from build123d import *

# Parameters (mm, degrees)
SKETCH1_W              = 25
SKETCH1_H              = 35
SKETCH1_R              = 3.45
SKETCH1_R_2            = 1.5
BOSS_EXTRUDE1_DEPTH    = 13
SKETCH5_W              = 21
SKETCH5_H              = 31
CUT_EXTRUDE1_DEPTH     = 11
CUT_EXTRUDE2_REACH     = 41.373
SKETCH7_R              = 2.5
BOSS_EXTRUDE3_DEPTH    = 13
SKETCH11_R             = 3.25
CUT_EXTRUDE4_DEPTH     = 12
CUT_EXTRUDE5_START     = 12
CUT_EXTRUDE5_OUTLINE_R = 1.75
CUT_EXTRUDE5_DEPTH     = 1


# Read off the part's stored shape, not the designer's step: Cut-Extrude5
with BuildPart() as part:
    # Sketch1 → Boss-Extrude1 (new body)
    with BuildSketch(Plane(origin=(0, 0, 0), x_dir=(1, 0, 0), z_dir=(0, 1, 0))):
        with Locations((0, -7.840328725)):
            Rectangle(SKETCH1_W, SKETCH1_H)
        with Locations(Location((0, 0, 0), (0, 0, 90))):
            Circle(SKETCH1_R, mode=Mode.SUBTRACT)
        with Locations(Location((8.5, 0, 0), (0, 0, 90))):
            Circle(SKETCH1_R_2, mode=Mode.SUBTRACT)
    extrude(amount=BOSS_EXTRUDE1_DEPTH)

    # Sketch5 → Cut-Extrude1 (cut)
    with BuildSketch(Plane(origin=(0, 13, 0), x_dir=(1, 0, 0), z_dir=(0, 1, 0))):
        with Locations((0, -7.840328725)):
            Rectangle(SKETCH5_W, SKETCH5_H)
    extrude(amount=-CUT_EXTRUDE1_DEPTH, mode=Mode.SUBTRACT)

    # Sketch7 → Cut-Extrude2 (cut, up to next)
    with BuildSketch(Plane.XY.offset(25.340328725), mode=Mode.PRIVATE) as cut_extrude2_sk1:
        with Locations((0, 7)):
            Circle(SKETCH7_R)
    cut_extrude2_tool1 = extrude(cut_extrude2_sk1.sketch, amount=-CUT_EXTRUDE2_REACH, mode=Mode.PRIVATE) & part.part
    add(cut_extrude2_tool1.solids().sort_by_distance((0, 7, 25.340329))[0], mode=Mode.SUBTRACT)

    # Sketch9 → Boss-Extrude3 (add, through all)
    with BuildSketch(Plane(origin=(0, 13, 0), x_dir=(1, 0, 0), z_dir=(0, 1, 0))):
        with BuildLine():
            Line((-16.5, 7.159671275), (-12.5, 7.159671275))
            Line((-12.5, 7.159671275), (-12.5, -2.840328725))
            Line((-12.5, -2.840328725), (-16.5, -2.840328725))
            ThreePointArc((-16.5, -2.840328725), (-21.5, 2.159671275), (-16.5, 7.159671275))
        make_face()
        with BuildLine():
            Line((-16.5, -7.804369497), (-12.5, -7.804369497))
            Line((-12.5, -7.804369497), (-12.5, -17.804369497))
            Line((-12.5, -17.804369497), (-16.5, -17.804369497))
            ThreePointArc((-16.5, -17.804369497), (-21.5, -12.804369497), (-16.5, -7.804369497))
        make_face()
        with BuildLine():
            Line((12.5, -7.804369497), (12.5, -17.804369497))
            Line((12.5, -17.804369497), (16.5, -17.804369497))
            ThreePointArc((16.5, -17.804369497), (21.5, -12.804369497), (16.5, -7.804369497))
            Line((16.5, -7.804369497), (12.5, -7.804369497))
        make_face()
        with BuildLine():
            Line((12.5, 7.159671275), (12.5, -2.840328725))
            Line((12.5, -2.840328725), (16.5, -2.840328725))
            ThreePointArc((16.5, -2.840328725), (21.5, 2.159671275), (16.5, 7.159671275))
            Line((16.5, 7.159671275), (12.5, 7.159671275))
        make_face()
    extrude(amount=-BOSS_EXTRUDE3_DEPTH)

    # Sketch11 → Cut-Extrude4 (cut)
    with BuildSketch(Plane.XZ):
        with Locations(Location((-16.5, 12.800328725, 0), (0, 0, 270))):
            Circle(SKETCH11_R)
        with Locations(Location((-16.5, -2.159671275, 0), (0, 0, 270))):
            Circle(SKETCH11_R)
        with Locations(Location((16.5, 12.800328725, 0), (0, 0, 270))):
            Circle(SKETCH11_R)
        with Locations(Location((16.5, -2.159671275, 0), (0, 0, 270))):
            Circle(SKETCH11_R)
    extrude(amount=-CUT_EXTRUDE4_DEPTH, mode=Mode.SUBTRACT)

    # Cut-Extrude5 outline → Cut-Extrude5 (cut)
    with BuildSketch(Plane(origin=(0, 0, 0), x_dir=(1, 0, 0), z_dir=(0, 1, 0)).offset(CUT_EXTRUDE5_START)):
        with Locations((-16.5, 2.159671275)):
            Circle(CUT_EXTRUDE5_OUTLINE_R)
        with Locations((16.5, -12.800328725)):
            Circle(CUT_EXTRUDE5_OUTLINE_R)
        with Locations((16.5, 2.159671275)):
            Circle(CUT_EXTRUDE5_OUTLINE_R)
        with Locations((-16.5, -12.800328725)):
            Circle(CUT_EXTRUDE5_OUTLINE_R)
    extrude(amount=CUT_EXTRUDE5_DEPTH, mode=Mode.SUBTRACT)


solid = part.part
Part model, mm, in its own coordinate system. A direction names the side the tool comes from. Give positions to 0.01 mm unless a question says otherwise; leave off trailing zeros. Order: outer loops, then holes, each group sorted by start corner. A loop starts at its lowest first (then second) coordinate and runs counter-clockwise, first axis right, second up. Notation, with made-up numbers: (-24, 69.5) - (-20, 69.5) arc R30 ccw to (-20, 102.5) - close; hole circle Ø8 at (-35.75, 29). An arc over 180 degrees is marked (long way). Use a Markdown table: item, result.
1) Flat gauge pins, fed straight in: P1, Ø7, axis at x = 17, z = 14.5, coming from the -Y side; P2, Ø3, axis at x = 15, y = 4.5, coming from the -Z side; P3, Ø2, axis at y = 5, z = 20.5, coming from the -X side; P4, Ø1, axis at x = 13.5, y = 10.5, coming from the +Z side. Where does each tip first touch, or does it go through?
Checked values:
| item | result |
|---|---|
| P1 | y = 0 |
| P2 | z = -7.16 |
| P3 | x = -12.5 |
| P4 | z = 17.8 |
2) 3-axis set-ups, long thin cutter, end or side, ignore diameter. For faces 5 (the flat face through (-12.5, 6, 5)), 6 (the flat face through (15, 7, 7.804)), 7 (the cylindrical face through (19.722, 5.916, 13.223)), 8 (the flat face through (14, 7, 17.804)): which of +Z, -Z, +X, -X, +Y, -Y reach the whole face in a straight line?
Checked values:
| item | result |
|---|---|
| face 5 | -X, +Y, -Y |
| face 6 | +X, +Y, -Y |
| face 7 | -Y |
| face 8 | +Z, +X, +Y, -Y |
3) Probe L1, parallel to Z at x = 4, y = 11.25; L2, parallel to X at y = 7.75, z = 12.5; L3, parallel to X at y = 10, z = 20.5. List the from-to ranges inside material, lowest first. Write a range as from..to.
Checked values:
| item | result |
|---|---|
| L1 | -9.66..-7.66, 23.34..25.34 |
| L2 | -21.49..-19.74, -13.26..-10.5, 10.5..13.26, 19.74..21.49 |
| L3 | -12.5..-10.5, 10.5..12.5 |
4) Saw through at D-D on y = 7. Count the separate pieces of the cut face and the enclosed holes in it, plus the area to 3 significant figures.
Checked values:
| item | result |
|---|---|
| separate pieces | 1 |
| enclosed holes | 4 |
| area | 398 mm² |
5) Saw through at B-B on x = 0. List the corners of the cut face in (y, z), plus the area to 3 significant figures.
Checked values:
| item | result |
|---|---|
| outline | (0, -9.66) - (13, -9.66) - (13, -7.66) - (2, -7.66) - (2, -3.45) - (0, -3.45) - close; (0, 3.45) - (2, 3.45) - (2, 23.34) - (4.5, 23.34) - (4.5, 25.34) - (0, 25.34) - close; (9.5, 23.34) - (13, 23.34) - (13, 25.34) - (9.5, 25.34) - close |
| area | 90.2 mm² |
6) Two-plate mould, pull along Z, no slides. Class faces 1 (the cylindrical face through (-21.5, 6.59, -2.05)), 2 (the flat face through (-14, 7, 17.804)), 3 (the cylindrical face through (10, 1, 0)), 4 (the flat face through (12.5, 6, 22)): +Z half, -Z half, draft (parallel to the pull), parting line (faces both ways), or undercut.
Checked values:
| item | result |
|---|---|
| face 1 | undercut |
| face 2 | +Z half |
| face 3 | undercut |
| face 4 | draft |
7) Saw through at C-C on z = 0.5. List the corners of the cut face in (x, y).
Checked values:
| item | result |
|---|---|
| outline | (-20.73, 0) - (-18.37, 0) - (-18.37, 12) - (-14.63, 12) - (-14.63, 0) - (-3.41, 0) - (-3.41, 2) - (-10.5, 2) - (-10.5, 13) - (-20.73, 13) - close; (3.41, 0) - (7.09, 0) - (7.09, 2) - (3.41, 2) - close; (9.91, 0) - (14.63, 0) - (14.63, 12) - (18.37, 12) - (18.37, 0) - (20.73, 0) - (20.73, 13) - (10.5, 13) - (10.5, 2) - (9.91, 2) - close |
8) Saw through at A-A on x = 8.5. List the corners of the cut face in (y, z).
Checked values:
| item | result |
|---|---|
| outline | (0, -9.66) - (13, -9.66) - (13, -7.66) - (2, -7.66) - (2, -1.5) - (0, -1.5) - close; (0, 1.5) - (2, 1.5) - (2, 23.34) - (13, 23.34) - (13, 25.34) - (0, 25.34) - close |
